The model under review builds one solid part; all positions refer to its coordinate system, in mm. Coordinates: 2 decimals unless noted, no trailing zeros. Write each loop counter-clockwise with the first axis right and the second up, starting at its lowest first coordinate (ties: lowest second). Pieces come first, ordered by that corner, then holes. Notation, with made-up numbers: (7, 73.25) -> (52, 73.25) arc R18 ccw to (52, 98.25) -> close; hole circle Ø8 at (-10.5, 39.5). An arc over 180 degrees is marked (long way). Write each question's results on one line, items separated by ' | '.
```python
from build123d import *

# Parameters (mm, degrees)
SKETCH1_R           = 10
SKETCH1_R_2         = 7.5
BOSS_EXTRUDE1_DEPTH = 0.25
SKETCH2_R           = 9.5
SKETCH2_R_2         = 7.5
BOSS_EXTRUDE2_DEPTH = 5
FILLET1_R           = 1


with BuildPart() as part:
    # Sketch1 → Boss-Extrude1 (new body)
    with BuildSketch(Plane(origin=(0, 0, 0), x_dir=(0, 0, -1), z_dir=(1, 0, 0))):
        Circle(SKETCH1_R)
        Circle(SKETCH1_R_2, mode=Mode.SUBTRACT)
    extrude(amount=BOSS_EXTRUDE1_DEPTH)

    # Sketch2 → Boss-Extrude2 (add)
    with BuildSketch(Plane(origin=(0.25, 0, 0), x_dir=(0, 0, -1), z_dir=(1, 0, 0))):
        Circle(SKETCH2_R)
        Circle(SKETCH2_R_2, mode=Mode.SUBTRACT)
    extrude(amount=BOSS_EXTRUDE2_DEPTH)

    # Fillet1
    fillet1_edges = [part.edges().sort_by_distance(p)[0] for p in [
        (5.25, 0, 9.5),
    ]]
    fillet(fillet1_edges, radius=FILLET1_R)


solid = part.part
```
Q1. Draft analysis for pull direction Z (two halves, no side actions). For faces 1 (the cylindrical face through (2.22, -8.43, -4.38)), 2 (the flat face through (0.25, -4, -9)), 3 (the cylindrical face through (2.588, 0.33, 7.493)), state which applies: pulls with the +Z half, pulls with the -Z half, needs draft (parallel to the pull), parting line crosses it, or undercut.
Solution:
face 1: parting line crosses it | face 2: needs draft | face 3: undercut
Q2. Add section C-C (x = 2.2). Write out the cut boundary in (y, z).
Solution:
outline: circle Ø19 at (0, 0); hole circle Ø15 at (0, 0)
Q3. For line 1 (Y direction, x = 1.1, z = 0); line 2 (Z direction, x = 0.9, y = 3.25); line 3 (Y direction, x = 1.6, z = -5.75), list the stretches that pass through material, from the lowest coordinate up. Write a range as from..to.
Solution:
line 1: -9.5..-7.5, 7.5..9.5 | line 2: -8.93..-6.76, 6.76..8.93 | line 3: -7.56..-4.82, 4.82..7.56
Q4. Clearance check with flat-ended pins moving along their axes: P1, Ø1.5, axis at y = 6, z = 0, coming from the -X side; P2, Ø1, axis at x = 3.5, z = 2.5, coming from the -Y side; P3, Ø3, axis at x = 4, y = 2.5, coming from the +Z side. State where each tip first meets the part, or that it passes through.
Solution:
P1: through | P2: y = -9.29 | P3: z = 9.45
Q5. Add section A-A (y = 0). Write out the cut boundary in (x, z).
Solution:
outline: (0, -10) -> (0.25, -10) -> (0.25, -9.5) -> (4.25, -9.5) arc R1 ccw to (5.25, -8.5) -> (5.25, -7.5) -> (0, -7.5) -> close; (0, 7.5) -> (5.25, 7.5) -> (5.25, 8.5) arc R1 ccw to (4.25, 9.5) -> (0.25, 9.5) -> (0.25, 10) -> (0, 10) -> close
